Geometry check sheet. Reference: the model listing, model coordinates, mm. Give positions to 0.01 mm unless a question says otherwise; leave off trailing zeros. Loops run counter-clockwise (first coordinate to the right, second up) from the corner with the lowest first, then second, coordinate; pieces in that order, holes last.
1. Go/stop test with flat-tipped pins: pin 1 Ø5 at (y, z) = (4, -9) entering from -X; pin 2 Ø6 at (y, z) = (13, 13.5) entering from -X; pin 3 Ø2 at (y, z) = (3.5, -2) entering from +X (3 decimals). Record where each tip stops, or that it passes through.
2. Cross-section at A-A, the plane y = 3.25. Record the cut outline in (x, z).
3. Cross-section at D-D, the plane z = 16.5. Record the cut outline in (x, y).
4. Cross-section at C-C, the plane x = 0. State how many separate pieces and enclosed holes the cut face has, plus the area to 3 significant figures.
5. Cross-section at B-B, the plane z = 1. Record the cut outline in (x, y), plus the area to 3 significant figures.
6. Material ranges on L1, parallel to Y at x = 0.5, z = -15; L2, parallel to Y at x = -14, z = 12.5; L3, parallel to Y at x = 3, z = -5.5, recorded low to high.
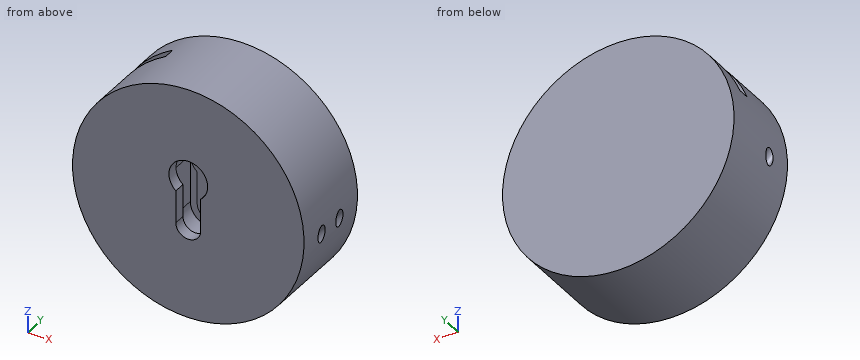
from build123d import *
from build123d.topology import SkipClean

# Parameters (mm, degrees)
SKETCH1_R               = 20
BOSS_EXTRUDE1_DEPTH     = 15
SKETCH2_R               = 3.35
CUT_EXTRUDE1_DEPTH      = 6
CUT_EXTRUDE2_START      = 4
CUT_EXTRUDE2_DEPTH      = 4
CUT_SWEEP1_PROFILE_R    = 1
CUT_SWEEP2_PROFILE_R    = 1
CUT_EXTRUDE3_DEPTH      = 1
CUT_EXTRUDE3_DEPTH_BACK = 1


with BuildPart() as part:
    # Sketch1 → Boss-Extrude1 (new body)
    with BuildSketch(Plane(origin=(0, 0, 0), x_dir=(1, 0, 0), z_dir=(0, 1, 0))):
        with Locations(Location((0, 0, 0), (0, 0, 270))):
            Circle(SKETCH1_R)
    extrude(amount=BOSS_EXTRUDE1_DEPTH)

    # Sketch2 → Cut-Extrude1 (cut)
    with BuildSketch(Plane.XZ):
        with Locations((0, 4.085684088)):
            Circle(SKETCH2_R)
        with BuildLine():
            Line((2.15, 4.085684088), (2.15, -4.085684088))
            ThreePointArc((2.15, -4.085684088), (0, -6.235684088), (-2.15, -4.085684088))
            Line((-2.15, -4.085684088), (-2.15, 4.085684088))
            ThreePointArc((-2.15, 4.085684088), (0, 6.235684088), (2.15, 4.085684088))
        make_face()
    extrude(amount=-CUT_EXTRUDE1_DEPTH, mode=Mode.SUBTRACT)

    # Sketch3 → Cut-Extrude2 (cut)
    with SkipClean():  # the faces are left unmerged after this step: merging them gives an invalid solid
        with BuildSketch(Plane.XZ.offset(-6).offset(CUT_EXTRUDE2_START)):
            with BuildLine():
                Line((-3.35, -4.085684088), (-3.35, 4.085684088))
                ThreePointArc((-3.35, 4.085684088), (0, 7.435684088), (3.35, 4.085684088))
                Line((3.35, 4.085684088), (3.35, -4.085684088))
                ThreePointArc((3.35, -4.085684088), (0, -7.435684088), (-3.35, -4.085684088))
            make_face()
        extrude(amount=-CUT_EXTRUDE2_DEPTH, mode=Mode.SUBTRACT)
    add(part.part.scale(1), mode=Mode.REPLACE)  # the faces are merged on a copy

    # Cut-Sweep1: sweep along a path in Sketch6
    with BuildLine(Plane(origin=(0, 10, 0), x_dir=(1, 0, 0), z_dir=(0, 1, 0))) as cut_sweep1_path:
        Line((32.713303623, -11.500100188), (10.606601718, 10.606601718))
        ThreePointArc((10.606601718, 10.606601718), (-5.740251485, 13.858192988), (-15, 0))
        Line((-15, 0), (-15, -54.761265519))
    # Cut-Sweep1 profile (on start of the path) → Cut-Sweep1 (sweep, cut)
    with BuildSketch(Plane(origin=(32.713303623, 10, 11.500100188), x_dir=(-0.7071067811865515, 0, 0.7071067811865437), z_dir=(-0.7071067811865437, 0, -0.7071067811865515))):
        Circle(CUT_SWEEP1_PROFILE_R)
    sweep(path=cut_sweep1_path.line, mode=Mode.SUBTRACT)

    # Cut-Sweep2: sweep along a path in Sketch5
    with BuildLine(Plane(origin=(0, 5, 0), x_dir=(-1, 0, 0), z_dir=(0, -1, 0))) as cut_sweep2_path:
        Line((-32.713303623, -11.500100188), (-10.606601718, 10.606601718))
        ThreePointArc((-10.606601718, 10.606601718), (0, 15), (10.606601718, 10.606601718))
        Line((10.606601718, 10.606601718), (41.577001277, -20.363797841))
    # Cut-Sweep2 profile (on start of the path) → Cut-Sweep2 (sweep, cut)
    with BuildSketch(Plane(origin=(32.713303623, 5, 11.500100188), x_dir=(-0.7071067811865515, 0, 0.7071067811865437), z_dir=(-0.7071067811865437, 0, -0.7071067811865515))):
        Circle(CUT_SWEEP2_PROFILE_R)
    sweep(path=cut_sweep2_path.line, mode=Mode.SUBTRACT)

    # Sketch19 → Cut-Extrude3 (cut, two sides: drawn at the far end of the back side and taken through both)
    with BuildSketch(Plane(origin=(0, 10, 0), x_dir=(1, 0, 0), z_dir=(0, 1, 0)).offset(-CUT_EXTRUDE3_DEPTH_BACK)):
        Polygon((-14.949747468, 5.870733518), (-14, 0), (-8.665269788, -20.660460329), (-22.201970025, -20.660460329), align=None)
    extrude(amount=CUT_EXTRUDE3_DEPTH + CUT_EXTRUDE3_DEPTH_BACK, mode=Mode.SUBTRACT)


solid = part.part
Result:
1. pin 1: stops at x = -18.91
1. pin 2: stops at x = -17.02
1. pin 3: stops at x = 19.975
2. outline: circle Ø40 at (0, 0); hole (-3.35, -4.09) arc R3.35 ccw to (3.35, -4.09) - (3.35, 4.09) arc R3.35 ccw to (-3.35, 4.09) - close
3. outline: (-11.3, 0) - (11.3, 0) - (11.3, 15) - (-11.3, 15) - (-11.3, 11) - (-9.74, 11) - (-9.74, 9) - (-11.3, 9) - close
4. separate pieces: 1
4. enclosed holes: 2
4. area: 507 mm2
5. outline: (-19.97, 0) - (-2.15, 0) - (-2.15, 2) - (-3.35, 2) - (-3.35, 6) - (3.35, 6) - (3.35, 2) - (2.15, 2) - (2.15, 0) - (19.97, 0) - (19.97, 15) - (-19.97, 15) - close; hole (-16.83, 9) - (-13.74, 9) - (-13.74, 11) - (-16.83, 11) - close
5. area: 558 mm2
6. L1: y = 0 to 4, 6 to 9, 11 to 15
6. L2: y = 0 to 9, 11 to 15
6. L3: y = 0 to 2, 6 to 15
